```python
from build123d import *

# Parameters (mm, degrees)
SKETCH_1_W          = 65
SKETCH_1_H          = 46
EXTRUDE_1_DEPTH     = 3
SKETCH_2_W          = 65
SKETCH_2_H          = 15
EXTRUDE_2_DEPTH     = 3
SKETCH_3_W          = 65
SKETCH_3_H          = 46
EXTRUDE_3_DEPTH     = 3
SKETCH_4_R          = 3
CUT_EXTRUDE_1_DEPTH = 83.35289916


with BuildPart() as part:
    # 草图1 → 凸台-拉伸1 (new body)
    with BuildSketch(Plane(origin=(0, 0, 0), x_dir=(1, 0, 0), z_dir=(0, 1, 0))):
        with Locations((32.5, 23)):
            Rectangle(SKETCH_1_W, SKETCH_1_H)
    extrude(amount=EXTRUDE_1_DEPTH)

    # 草图2 → 凸台-拉伸2 (add)
    with BuildSketch(Plane.XY):
        with Locations((32.5, 10.5)):
            Rectangle(SKETCH_2_W, SKETCH_2_H)
    extrude(amount=-EXTRUDE_2_DEPTH)

    # 草图3 → 凸台-拉伸3 (add)
    with BuildSketch(Plane(origin=(0, 18, 0), x_dir=(1, 0, 0), z_dir=(0, 1, 0))):
        with Locations((32.5, 23)):
            Rectangle(SKETCH_3_W, SKETCH_3_H)
    extrude(amount=EXTRUDE_3_DEPTH)

    # 草图4 → 切除-拉伸1 (cut, through all)
    with BuildSketch(Plane.XZ):
        with Locations(Location((32.5, -23, 0), (0, 0, 270))):
            Circle(SKETCH_4_R)
        with Locations(Location((55, -34, 0), (0, 0, 270))):
            Circle(SKETCH_4_R)
        with Locations(Location((55, -12, 0), (0, 0, 270))):
            Circle(SKETCH_4_R)
        with Locations(Location((10, -34, 0), (0, 0, 270))):
            Circle(SKETCH_4_R)
        with Locations(Location((10, -12, 0), (0, 0, 270))):
            Circle(SKETCH_4_R)
    extrude(amount=-CUT_EXTRUDE_1_DEPTH, mode=Mode.SUBTRACT)


solid = part.part
```
Can you work these out from the model? Positions are in its coordinate system, mm. A direction names the side the tool comes from. Give positions to 0.01 mm unless a question says otherwise; leave off trailing zeros. Loops run counter-clockwise (first coordinate to the right, second up) from the corner with the lowest first, then second, coordinate; pieces in that order, holes last. Notation, with made-up numbers: M -38,-26 L -11,-26 A27 cw -11,-8 Z; hole C -31.75,87 d10. An arc over 180 degrees is marked long. One line per question, with ' | ' between items. Start each with the question number.
Q1. If we section it at D-D (x = 32.5): Please give me the cut outline in (y, z), plus the area to 3 significant figures.
Q2. If we section it at C-C (z = -34): Please give me the cut outline in (x, y).
Q3. If we section it at A-A (z = -17): Please give me the cut outline in (x, y), plus the area to 3 significant figures.
Q4. If we section it at B-B (y = 2): Please give me the cut outline in (x, z).
Q5. If I drill on line 1 (X direction, y = 20, z = -34); line 2 (Y direction, x = 39, z = -37); line 3 (X direction, y = 2.75, z = -14), over which ranges is the centre line in solid material (lowest first)? Write a range as from..to.
Q6. For pin 1 Ø7 at (x, z) = (10, -34) entering from +Y, with a flat end and sliding along its axis, tell me the tip position at first contact or that it passes through.
Q7. If we mould it in two halves opening along Z, with no side actions, what happens to faces 3 (the flat face through (32, 19, -46)), 4 (the cylindrical face through (10, 19, -9)), 5 (the flat face through (32, 21, -18))? For each: +Z half, -Z half, draft (parallel to the pull), parting line (faces both ways), or undercut.
Q8. For faces 1 (the flat face through (32, 10, 0)), 2 (the flat face through (32, 3, -30)), which set-ups out of +Z, -Z, +X, -X, +Y, -Y let a thin tool reach every point of the face, with its end or its side?
Computed:
1) outline: M 0,-46 L 3,-46 L 3,-26 L 0,-26 Z; M 0,-20 L 3,-20 L 3,-3 L 18,-3 L 18,-20 L 21,-20 L 21,0 L 0,0 Z; M 18,-46 L 21,-46 L 21,-26 L 18,-26 Z | area: 285 mm²
2) outline: M 0,0 L 7,0 L 7,3 L 0,3 Z; M 0,18 L 7,18 L 7,21 L 0,21 Z; M 13,0 L 52,0 L 52,3 L 13,3 Z; M 13,18 L 52,18 L 52,21 L 13,21 Z; M 58,0 L 65,0 L 65,3 L 58,3 Z; M 58,18 L 65,18 L 65,21 L 58,21 Z
3) outline: M 0,0 L 65,0 L 65,3 L 0,3 Z; M 0,18 L 65,18 L 65,21 L 0,21 Z | area: 390 mm²
4) outline: M 0,-46 L 65,-46 L 65,0 L 0,0 Z; hole C 10,-34 d6; hole C 10,-12 d6; hole C 32.5,-23 d6; hole C 55,-34 d6; hole C 55,-12 d6
5) line 1: x = 0..7, 13..52, 58..65 | line 2: y = 0..3, 18..21 | line 3: x = 0..7.76, 12.24..52.76, 57.24..65
6) pin 1: stops at y = 21
7) face 3: -Z half | face 4: undercut | face 5: draft
8) face 1: +Z, +X, -X, +Y, -Y | face 2: -Z, +X, -X
